Here's the drawing with two shaded views (mm, measured from the low corner). I have some questions. Give positions to 0.01 mm unless a question says otherwise; leave off trailing zeros. Order: outer loops, then holes, each group sorted by start corner. A loop starts at its lowest first (then second) coordinate and runs counter-clockwise, first axis right, second up. Notation, with made-up numbers: M 8.25,52 L 36.25,52 A22 ccw 36.25,74 Z; hole C 63.5,47 d3. An arc over 180 degrees is marked long. Use a Markdown table: item, result. Add a question column.
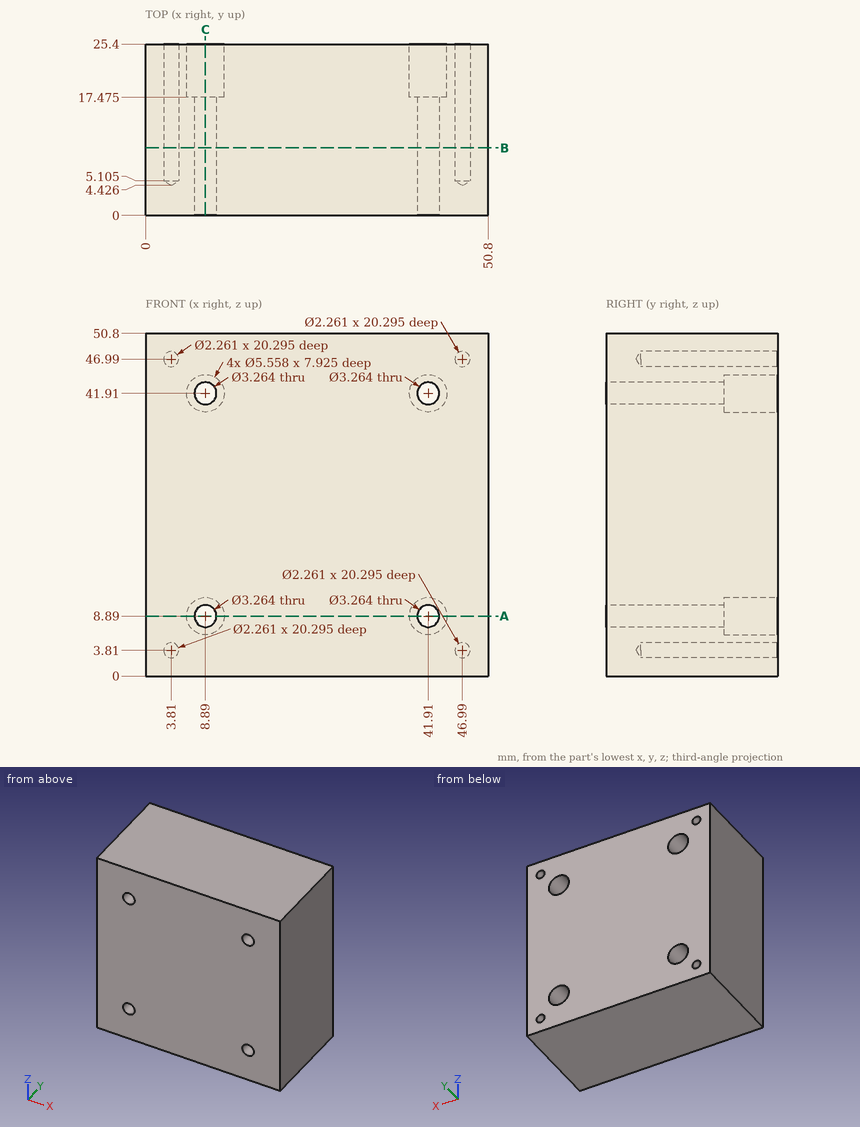
1) Please list where these lines run through material, in increasing order: line 1 (Z direction, x = 42, y = 17); line 2 (X direction, y = 21, z = 8.89); line 3 (X direction, y = 17.25, z = 46.99). Write a range as from..to.
2) Suppose I cut it at C-C on x = 8.89. Please give me the cut outline in (y, z) (1 decimal).
3) Suppose I cut it at B-B on y = 10. Count the separate pieces of the cut face and the enclosed holes in it, and give its area (3 significant figures).
4) For pin 1 (3.5 mm diameter, centred on x = 41.91, z = 8.89, fed in from +Y) (1 decimal); pin 2 (1.7 mm diameter, centred on x = 8.5, z = 42.5, fed in from +Y); pin 3 (1.8 mm diameter, centred on x = 46.99, z = 3.81, fed in from +Y), each with a flat end and sliding along its axis, tell me the tip position at first contact or that it passes through.
5) Suppose I cut it at A-A on z = 8.89. Please give me the cut outline in (x, y) (1 decimal).
Values found:
| question | item | result |
|---|---|---|
| 1 | line 1 | z = 0..7.26, 10.52..40.28, 43.54..50.8 |
| 1 | line 2 | x = 0..6.11, 11.67..39.13, 44.69..50.8 |
| 1 | line 3 | x = 0..2.68, 4.94..45.86, 48.12..50.8 |
| 2 | outline | M 0,0 L 25.4,0 L 25.4,6.1 L 17.5,6.1 L 17.5,7.3 L 0,7.3 Z; M 0,10.5 L 17.5,10.5 L 17.5,11.7 L 25.4,11.7 L 25.4,39.1 L 17.5,39.1 L 17.5,40.3 L 0,40.3 Z; M 0,43.5 L 17.5,43.5 L 17.5,44.7 L 25.4,44.7 L 25.4,50.8 L 0,50.8 Z |
| 3 | separate pieces | 1 |
| 3 | enclosed holes | 8 |
| 3 | area | 2,530 mm^2 |
| 4 | pin 1 | stops at y = 17.5 |
| 4 | pin 2 | passes through |
| 4 | pin 3 | stops at y = 4.97 |
| 5 | outline | M 0,0 L 7.3,0 L 7.3,17.5 L 6.1,17.5 L 6.1,25.4 L 0,25.4 Z; M 10.5,0 L 40.3,0 L 40.3,17.5 L 39.1,17.5 L 39.1,25.4 L 11.7,25.4 L 11.7,17.5 L 10.5,17.5 Z; M 43.5,0 L 50.8,0 L 50.8,25.4 L 44.7,25.4 L 44.7,17.5 L 43.5,17.5 Z |
